Verification items for the finished model (mm, model axes). A direction names the side the tool comes from. Coordinates: 2 decimals unless noted, no trailing zeros. Write each loop counter-clockwise with the first axis right and the second up, starting at its lowest first coordinate (ties: lowest second). Pieces come first, ordered by that corner, then holes. Notation, with made-up numbers: (34.25, 62.25) -> (49.25, 62.25) arc R14 cw to (49.25, 69.25) -> close; hole circle Ø9 at (-40, 42.5). An arc over 180 degrees is marked (long way). Write item = value, one per line. Start each with the question number.
(1) Section check A-A (y = 0.75). Record the cut outline in (x, z).
(2) Section check B-B (z = 15). Record the cut outline in (x, y).
(3) Gauge pin test, flat ends, axial feed: pin 1 Ø2 at (x, z) = (-1.5, 28.5) entering from +Y; pin 2 Ø2.5 at (x, z) = (0, 35) entering from +Y. Record the tip position at first contact, or that the pin passes through.
(4) Mould release check, pull along Z, two halves, no side actions. Record for faces 3 (the face through (-1, -1, 0)), 4 (the face through (-0.325, -6.486, 33.536)), 5 (the face through (-0.27, -1.22, 0.86)): released by +Z, released by -Z, zero draft, split by the parting line, or undercut.
(5) Section check D-D (x = 0). Record the cut outline in (y, z), plus the area to 3 significant figures.
(6) Section check C-C (y = -6.25). Record the cut outline in (x, z).
(7) Set-up check for faces 1 (the face through (-1.5, -6.49, 5.07)), 2 (the face through (0, -5.5, 20)): record each of +Z, -Z, +X, -X, +Y, -Y from which the full face is reachable in a straight line by a thin tool's end or side.
(8) Material ranges on probe 1 along Z at (x, y) = (0, -6.3); probe 2 along Y at (x, z) = (2, 31); probe 3 along Z at (x, y) = (2.5, 3.5), recorded low to high. Write a range as [from, to].
```python
from build123d import *

# Parameters (mm, degrees)
SKETCH_W     = 7.5
SKETCH_H     = 11
SKETCH_R     = 1.25
PAD_DEPTH    = 1.75
SKETCH001_W  = 7.5
SKETCH001_H  = 38.5
SKETCH001_R  = 1.5
PAD001_DEPTH = 2


with BuildPart() as part:
    # Sketch → Pad (new body)
    with BuildSketch(Plane.XY):
        Rectangle(SKETCH_W, SKETCH_H)
        Circle(SKETCH_R, mode=Mode.SUBTRACT)
    extrude(amount=PAD_DEPTH)

    # Sketch001 (on Face3 of Pad) → Pad001 (join)
    with BuildSketch(Plane.XZ.offset(5.5)):
        with Locations((0, 19.25)):
            Rectangle(SKETCH001_W, SKETCH001_H)
        with Locations((0, 5)):
            Circle(SKETCH001_R, mode=Mode.SUBTRACT)
        with Locations((0, 15)):
            Circle(SKETCH001_R, mode=Mode.SUBTRACT)
        with Locations((0, 25)):
            Circle(SKETCH001_R, mode=Mode.SUBTRACT)
        with Locations((0, 35)):
            Circle(SKETCH001_R, mode=Mode.SUBTRACT)
    extrude(amount=PAD001_DEPTH)


solid = part.part
```
Response:
q1.outline = (-3.75, 0) -> (-1, 0) -> (-1, 1.75) -> (-3.75, 1.75) -> close; (1, 0) -> (3.75, 0) -> (3.75, 1.75) -> (1, 1.75) -> close
q2.outline = (-3.75, -7.5) -> (-1.5, -7.5) -> (-1.5, -5.5) -> (-3.75, -5.5) -> close; (1.5, -7.5) -> (3.75, -7.5) -> (3.75, -5.5) -> (1.5, -5.5) -> close
q3.pin_1 = -5.5
q3.pin_2 = through
q4.face_3 = released by -Z
q4.face_4 = undercut
q4.face_5 = zero draft
q5.outline = (-7.5, 0) -> (-1.25, 0) -> (-1.25, 1.75) -> (-5.5, 1.75) -> (-5.5, 3.5) -> (-7.5, 3.5) -> close; (-7.5, 6.5) -> (-5.5, 6.5) -> (-5.5, 13.5) -> (-7.5, 13.5) -> close; (-7.5, 16.5) -> (-5.5, 16.5) -> (-5.5, 23.5) -> (-7.5, 23.5) -> close; (-7.5, 26.5) -> (-5.5, 26.5) -> (-5.5, 33.5) -> (-7.5, 33.5) -> close; (-7.5, 36.5) -> (-5.5, 36.5) -> (-5.5, 38.5) -> (-7.5, 38.5) -> close; (1.25, 0) -> (5.5, 0) -> (5.5, 1.75) -> (1.25, 1.75) -> close
q5.area = 67.9 mm2
q6.outline = (-3.75, 0) -> (3.75, 0) -> (3.75, 38.5) -> (-3.75, 38.5) -> close; hole circle Ø3 at (0, 5); hole circle Ø3 at (0, 15); hole circle Ø3 at (0, 25); hole circle Ø3 at (0, 35)
q7.face_1 = +Y, -Y
q7.face_2 = +Z, +X, -X, +Y
q8.probe_1 = [0, 3.5], [6.5, 13.5], [16.5, 23.5], [26.5, 33.5], [36.5, 38.5]
q8.probe_2 = [-7.5, -5.5]
q8.probe_3 = [0, 1.75]
